Check sheet for the modelled part. Datum: model origin and axes. Units: mm. Face numbers are marked on the shaded views. Round coordinates to 2 decimals unless told otherwise and drop trailing zeros. Loops run counter-clockwise (first coordinate to the right, second up) from the corner with the lowest first, then second, coordinate; pieces in that order, holes last. Notation, with made-up numbers: (86, 6.5) - (101, 6.5) arc R29 cw to (101, 39.5) - close; hole circle Ø6 at (25.5, -24). An arc over 180 degrees is marked (long way). Return JSON: item names as keys, results as strings.
from build123d import *

# Parameters (mm, degrees)
SKETCH1_W           = 212
SKETCH1_H           = 162
SKETCH1_W_2         = 206
SKETCH1_H_2         = 156
SKETCH1_W_3         = 200
SKETCH1_H_3         = 150
BOSS_EXTRUDE1_DEPTH = 100
SKETCH1_4_W         = 212
SKETCH1_4_H         = 162
SKETCH1_4_W_2       = 206
SKETCH1_4_H_2       = 156
CUT_EXTRUDE2_DEPTH  = 10
SKETCH2_5_R         = 1.5
SKETCH2_5_R_2       = 6
CUT_EXTRUDE3_DEPTH  = 6
SKETCH2_W           = 10
SKETCH2_H           = 5.5
SKETCH2_R           = 1.5
BOSS_EXTRUDE4_DEPTH = 10.5
CHAMFER1_SIZE       = 2
BOSS_EXTRUDE5_START = 3
SKETCH2_12_W        = 22.5
SKETCH2_12_H        = 36.742349428
SKETCH2_12_R        = 6
SKETCH2_12_R_2      = 1.5
BOSS_EXTRUDE5_DEPTH = 3
SKETCH2_13_R        = 1.5
SKETCH2_13_R_2      = 3
CUT_EXTRUDE6_DEPTH  = 6
SKETCH2_14_R        = 2.5
SKETCH2_14_R_2      = 1.5
CUT_EXTRUDE7_DEPTH  = 3
SKETCH2_18_R        = 1.4
SKETCH2_18_W        = 7
SKETCH2_18_H        = 7
BOSS_EXTRUDE7_DEPTH = 15
BOSS_EXTRUDE8_DEPTH = 15
SKETCH13_R          = 1.4
SKETCH13_R_2        = 1.5
CUT_EXTRUDE14_DEPTH = 7


with BuildPart() as part:
    # Sketch1 → Boss-Extrude1 (new body)
    # profile 1 of 2: a face of its own
    with BuildSketch(Plane.XY):
        Rectangle(SKETCH1_W, SKETCH1_H)
        Rectangle(SKETCH1_W_2, SKETCH1_H_2, mode=Mode.SUBTRACT)
    # profile 2 of 2: a face of its own
    with BuildSketch(Plane.XY):
        Rectangle(SKETCH1_W_2, SKETCH1_H_2)
        Rectangle(SKETCH1_W_3, SKETCH1_H_3, mode=Mode.SUBTRACT)
    extrude(amount=BOSS_EXTRUDE1_DEPTH)

    # Sketch1<4> → Cut-Extrude2 (cut)
    with BuildSketch(Plane.XY):
        Rectangle(SKETCH1_4_W, SKETCH1_4_H)
        Rectangle(SKETCH1_4_W_2, SKETCH1_4_H_2, mode=Mode.SUBTRACT)
    extrude(amount=CUT_EXTRUDE2_DEPTH, mode=Mode.SUBTRACT)

    # Sketch2<5> → Cut-Extrude3 (cut)
    with BuildSketch(Plane.ZY.offset(106)):
        with Locations((40.75, -20.742349428)):
            Circle(SKETCH2_5_R)
        with Locations((59.25, -20.742349428)):
            Circle(SKETCH2_5_R)
        with Locations((50, 0)):
            Circle(SKETCH2_5_R_2)
    extrude(amount=-CUT_EXTRUDE3_DEPTH, mode=Mode.SUBTRACT)

    # Sketch2 → Boss-Extrude4 (add)
    with BuildSketch(Plane.ZY.offset(106)):
        with Locations((50, 13.75)):
            Rectangle(SKETCH2_W, SKETCH2_H)
        with Locations(Location((50, 13.5, 0), (0, 0, 180))):
            Circle(SKETCH2_R, mode=Mode.SUBTRACT)
    extrude(amount=BOSS_EXTRUDE4_DEPTH)

    # Chamfer1
    chamfer1_edges = [part.edges().sort_by_distance(p)[0] for p in [
        (-116.5, 13.75, 55),
        (-116.5, 13.75, 45),
    ]]
    chamfer(chamfer1_edges, length=CHAMFER1_SIZE)

    # Sketch2<12> → Boss-Extrude5 (add)
    with BuildSketch(Plane.ZY.offset(106).offset(BOSS_EXTRUDE5_START)):
        with Locations((50, -7.371174714)):
            Rectangle(SKETCH2_12_W, SKETCH2_12_H)
        with Locations((50, 0)):
            Circle(SKETCH2_12_R, mode=Mode.SUBTRACT)
        with Locations((40.75, -20.742349428)):
            Circle(SKETCH2_12_R_2, mode=Mode.SUBTRACT)
        with Locations((59.25, -20.742349428)):
            Circle(SKETCH2_12_R_2, mode=Mode.SUBTRACT)
    extrude(amount=-BOSS_EXTRUDE5_DEPTH)

    # Sketch2<13> → Cut-Extrude6 (cut)
    with BuildSketch(Plane.ZY.offset(106)):
        with Locations((90, 0)):
            Circle(SKETCH2_13_R)
        with Locations((90, 27)):
            Circle(SKETCH2_13_R)
        with Locations((90, -27)):
            Circle(SKETCH2_13_R)
        with Locations((80, 0)):
            Circle(SKETCH2_13_R_2)
    extrude(amount=-CUT_EXTRUDE6_DEPTH, mode=Mode.SUBTRACT)

    # Sketch2<14> → Cut-Extrude7 (cut)
    # profile 1 of 5: a face of its own
    with BuildSketch(Plane.ZY.offset(106)):
        with Locations((90, 27)):
            Circle(SKETCH2_14_R)
        with Locations((90, 27)):
            Circle(SKETCH2_14_R_2, mode=Mode.SUBTRACT)
    # profile 2 of 5: a face of its own
    with BuildSketch(Plane.ZY.offset(106)):
        with Locations((90, 0)):
            Circle(SKETCH2_14_R)
        with Locations((90, 0)):
            Circle(SKETCH2_14_R_2, mode=Mode.SUBTRACT)
    # profile 3 of 5: a face of its own
    with BuildSketch(Plane.ZY.offset(106)):
        with Locations((90, -27)):
            Circle(SKETCH2_14_R)
        with Locations((90, -27)):
            Circle(SKETCH2_14_R_2, mode=Mode.SUBTRACT)
    # profile 4 of 5: a face of its own
    with BuildSketch(Plane.ZY.offset(106)):
        with BuildLine():
            ThreePointArc((92.5, 0), (90, 2.5), (87.5, 0))
            Line((87.5, 0), (88.5, 0))
            ThreePointArc((88.5, 0), (90, 1.5), (91.5, 0))
            Line((91.5, 0), (92.5, 0))
        make_face()
    # profile 5 of 5: a face of its own
    with BuildSketch(Plane.ZY.offset(106)):
        with BuildLine():
            Line((88.5, 0), (87.5, 0))
            ThreePointArc((87.5, 0), (90, -2.5), (92.5, 0))
            Line((92.5, 0), (91.5, 0))
            ThreePointArc((91.5, 0), (90, -1.5), (88.5, 0))
        make_face()
    extrude(amount=-CUT_EXTRUDE7_DEPTH, mode=Mode.SUBTRACT)

    # Sketch2<18> → Boss-Extrude7 (add)
    # profile 1 of 4: a face of its own
    with BuildSketch(Plane.ZY.offset(106)):
        Polygon((93, 88), (83, 81), (93, 81), (100, 81), (100, 88), align=None)
        with Locations((96.5, 84.5)):
            Circle(SKETCH2_18_R, mode=Mode.SUBTRACT)
    # profile 2 of 4: a face of its own
    with BuildSketch(Plane.ZY.offset(106)):
        with Locations((13.5, 84.5)):
            Rectangle(SKETCH2_18_W, SKETCH2_18_H)
        with Locations((13.5, 84.5)):
            Circle(SKETCH2_18_R, mode=Mode.SUBTRACT)
    # profile 3 of 4: a face of its own
    with BuildSketch(Plane.ZY.offset(106)):
        with Locations((13.5, -84.5)):
            Rectangle(SKETCH2_18_W, SKETCH2_18_H)
        with Locations((13.5, -84.5)):
            Circle(SKETCH2_18_R, mode=Mode.SUBTRACT)
    # profile 4 of 4: a face of its own
    with BuildSketch(Plane.ZY.offset(106)):
        Polygon((93, -81), (83, -81), (93, -88), (100, -88), (100, -81), align=None)
        with Locations((96.5, -84.5)):
            Circle(SKETCH2_18_R, mode=Mode.SUBTRACT)
    extrude(amount=-BOSS_EXTRUDE7_DEPTH)

    # Sketch12 → Boss-Extrude8 (add)
    with BuildSketch(Plane(origin=(106, 0, 0), x_dir=(0, 0, -1), z_dir=(1, 0, 0))):
        Polygon((-100, -81), (-100, -88), (-93, -88), (-83, -81), align=None)
        Polygon((-100, 81), (-100, 88), (-93, 88), (-83, 81), align=None)
    extrude(amount=-BOSS_EXTRUDE8_DEPTH)

    # Sketch13 → Cut-Extrude14 (cut)
    with BuildSketch(Plane.XY.offset(100)):
        with Locations((-95, 84.5)):
            Circle(SKETCH13_R)
        with Locations((-95, -84.5)):
            Circle(SKETCH13_R)
        with Locations((102, 84.5)):
            Circle(SKETCH13_R_2)
        with Locations(Location((102, -84.5, 0), (0, 0, 180))):
            Circle(SKETCH13_R_2)
    extrude(amount=-CUT_EXTRUDE14_DEPTH, mode=Mode.SUBTRACT)


solid = part.part
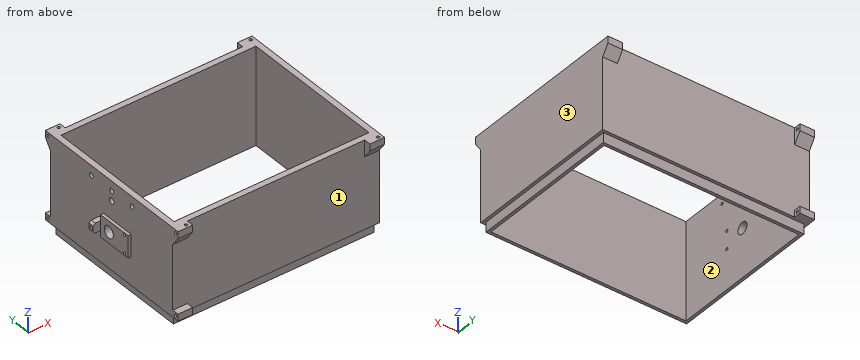
Q1. Draft check along X on the marked faces 1, 2 and 3. Enter one of: released by +X, released by -X, zero draft, split by the parting line, or undercut.
Answer key:
{"face 1": "undercut", "face 2": "undercut", "face 3": "released by +X"}
Q2. Sectioned sample at A-A (y = 48). Enter the section's corners in (x, z), plus the area to 3 significant figures.
Answer key:
{"outline": "(-106, 10) - (-103, 10) - (-103, 0) - (-100, 0) - (-100, 100) - (-106, 100) - close; (100, 0) - (103, 0) - (103, 10) - (106, 10) - (106, 100) - (100, 100) - close", "area": "1,140 mm²"}
Q3. Depth check by flat-ended pin: P1, Ø3, axis at x = -21, z = 15, coming from the +Y side; P2, Ø3.5, axis at y = 13.5, z = 50, coming from the -X side; P3, Ø5, axis at x = 4.5, z = 2.5, coming from the -Y side; P4, Ø0.8, axis at x = -94.5, y = 84, coming from the +Z side. Enter the tip coordinate at first touch or a pass-through.
Answer key:
{"P1": "stops at y = 81", "P2": "stops at x = -116.5", "P3": "stops at y = -78", "P4": "stops at z = 93"}
Q4. Scan lines: probe 1 along Z at (x, y) = (-102, -84.5); probe 2 along Y at (x, z) = (-95, 94); probe 3 along X at (y, z) = (84.5, 95.65). Record each from-to range of solid material in increasing order. Write a range as [from, to].
Answer key:
{"probe 1": "z = [10, 12.1], [14.9, 17], [88, 95.1], [97.9, 100]", "probe 2": "y = [-88, -85.9], [-83.1, -75], [75, 83.1], [85.9, 88]", "probe 3": "x = [91, 100.5], [103.5, 106]"}
Q5. Sectioned sample at B-B (z = 80). Enter the section's corners in (x, y).
Answer key:
{"outline": "(-106, -81) - (106, -81) - (106, 81) - (-106, 81) - (-106, 3) - (-100, 3) - (-100, 75) - (100, 75) - (100, -75) - (-100, -75) - (-100, -3) - (-106, -3) - close"}
